The model under review builds one solid part; all positions refer to its coordinate system, in mm. A direction names the side the tool comes from. Coordinates: 2 decimals unless noted, no trailing zeros. Write each loop counter-clockwise with the first axis right and the second up, starting at its lowest first coordinate (ties: lowest second). Pieces come first, ordered by that corner, then holes. Notation, with made-up numbers: M -39.5,2 L -11.5,2 A15 ccw -11.5,29 Z; hole C 41.5,14 d10. An arc over 180 degrees is marked long. Answer as a JSON object with one key per item and string values.
Autodesk Inventor part; units mm, degrees
ref_plane "Arbeitsebene1" through (17.5, 0, 0) normal (1, 0, 0) x (0, 1, 0)
ref_plane "Arbeitsebene3" through (40, 196, 0) normal (0, 1, 0) x (-1, 0, 0)
ref_plane "XY Plane" through (0, 0, 0) normal (0, 0, 1) x (1, 0, 0)
sketch "Skizze6" plane through (0, 0, 0) normal (0, 0, 1) x (0, 1, 0)
  line L0 (0, 181.4954) -> (0, -165.4211)
  line L1 (196, 0) -> (196, -80)
  line L2 (179, -27) -> (179, -63)
  arc A0 (191, 0) -> (179, -27) centre (215.375, -27) ccw
  arc A1 (179, -63) -> (196, -80) centre (196, -63) ccw
  line L3 (191, 0) -> (196, 0)
  line L4 (258.45, 0) -> (-43.075, 0)
  point P0 (0, 0)
  dimension "d29" = 80
  dimension "d30" = 392
  dimension "d31" = 358
  dimension "d32" = 5
  dimension "d35" = 27
revolve "Umdrehung1" add sketch "Skizze6" angle 89.4 mid plane about axis through (-181.4954, 0, 0) along (1, 0, 0)
ref_plane "Arbeitsebene1" through (17.5, 0, 0) normal (1, 0, 0) x (0, 1, 0)
sketch "Skizze7" plane through (17.5, 0, 0) normal (1, 0, 0) x (0, 1, 0)
  line L0 (0, 0) -> (200, 159.0872)
  line L1 (-40, 0) -> (240, 0)
  arc A0 (139.3167, -137.8654) -> (139.3167, 137.8654) centre (0, 0) ccw
  line L2 (153.3912, 122.0129) -> (151.3992, 124.5172)
  line L3 (151.3992, 124.5172) -> (149.8339, 123.2722)
  line L4 (149.8339, 123.2722) -> (149.3359, 123.8983)
  line L5 (149.3359, 123.8983) -> (137.5618, 114.5327)
  arc A1 (127.2331, -125.9077) -> (127.2331, 125.9077) centre (0, 0) ccw
  line L6 (137.5618, 114.5327) -> (140.0519, 111.4023)
  arc A2 (139.3167, -137.8654) -> (139.3167, 137.8654) centre (0, 0) ccw
  point P0 (140.0869, 111.4301)
  point P1 (151.3787, 124.501)
  point P2 (153.3912, 122.0129)
  point P3 (153.3912, 122.0129)
  dimension "d37" = 38.5
  dimension "d38" = 200
  dimension "d39" = 6.4
  dimension "d40" = 8
  dimension "d41" = 2
revolve "Umdrehung2" cut sketch "Skizze7" angle 360 about axis through (17.5, 0, 0) along (0, 0.7826082, 0.6225146) contours A1 L5 L4 L3 A0 L0 | A0 L3 L2
sketch "Skizze8" plane through (17.5, 151.826, 120.7678) normal (0, -0.7826082, -0.6225146) x (1, 0, 0)
  line L0 (-5.2, -3.0022) -> (-5.2, 3.0022)
  line L1 (-5.2, 3.0022) -> (0, 6.0044)
  line L2 (0, 6.0044) -> (5.2, 3.0022)
  line L3 (5.2, 3.0022) -> (5.2, -3.0022)
  line L4 (5.2, -3.0022) -> (0, -6.0044)
  line L5 (0, -6.0044) -> (-5.2, -3.0022)
  line L6 (0, 80.4096) -> (0, -281.6269)
  circle A0 centre (0, 0) radius 3.2
  line L7 (5.2, 3.0022) -> (10.4, 0)
  line L8 (10.4, 0) -> (5.2, -3.0022)
  point P0 (-17.5, 0)
  point P1 (0, 0)
  dimension "d43" = 10.4
extrude "Extrusion6" cut sketch "Skizze8" along normal through all contours L0 L1 L6 A0 L5 | L6 A0 L2 L3 L4 | L3 L7 L8
mirror "Spiegeln2" about plane through (0, 0, 0) normal (0, 0, 1) of "Extrusion6", "Umdrehung2"
ref_plane "Arbeitsebene3" through (40, 196, 0) normal (0, 1, 0) x (-1, 0, 0)
properties part number "Ventilator_Flansch_Oben"
(1) Wall thickness on line 1 along Z through (x, y) = (72, 150.5); line 2 along Z through (x, y) = (67, 135); line 3 along Y through (x, z) = (50, 77): over which ranges is each line inside the solid? List them lowest first. Write a range as from..to.
Results list:
{"line 1": "-125.56..-101.59, 101.59..125.56", "line 2": "-133.59..-118.27, 118.27..133.59", "line 3": "161.59..180.24"}
(2) Add section A-A on x = 37. Give the boundary of the cut face in (y, z), and give its area (3 significant figures).
Results list:
{"outline": "M 127.23,-125.91 L 139.32,-137.87 A196 ccw 139.32,137.87 L 127.23,125.91 A179 cw Z", "area": "4,970 mm²"}
(3) For pin 1 Ø3 at (y, z) = (177, 54) entering from +X; pin 2 Ø10 at (x, z) = (54.5, -103) entering from +Y; pin 3 Ø8 at (x, y) = (43.5, 156.5) entering from -Z, all flat-tipped, find the tip position at first contact; note any pin that passes through.
Results list:
{"pin 1": "x = 77.13", "pin 2": "y = 169.74", "pin 3": "z = -123.12"}
(4) Draft analysis for pull direction Y (two halves, no side actions). For faces 3 (the face through (19.447, 154.178, 119.394)), 4 (the face through (45.25, 178.99, -1.96)), state which applies: released by +Y, released by -Y, zero draft, split by the parting line, or undercut.
Results list:
{"face 3": "undercut", "face 4": "released by -Y"}
(5) For faces 1 (the face through (39.44, 133.19, -131.8)), 2 (the face through (14.864, 149.277, -113.013)), list the 3-axis set-ups (+Z, -Z, +X, -X, +Y, -Y) from which the entire face can be reached by the end or side of a thin tool; tool diameter is ignored.
Results list:
{"face 1": "-Z, +X, -X, -Y", "face 2": "none"}
